Model file for the job. Use its own axes, mm. Round coordinates to 2 decimals unless told otherwise and drop trailing zeros. Write each loop counter-clockwise with the first axis right and the second up, starting at its lowest first coordinate (ties: lowest second). Pieces come first, ordered by that corner, then holes. Notation, with made-up numbers: (-26.75, 43.5) - (15.25, 43.5) arc R24 ccw to (15.25, 67.5) - close; hole circle Ø8 at (23.25, -29.75). An arc over 180 degrees is marked (long way). Answer as a JSON object with one key per item and string values. Group by question number.
from build123d import *

# Parameters (mm, degrees)
SKETCH_1_R          = 1.9
EXTRUDE_1_DEPTH     = 72
SKETCH_2_R          = 2.25
CUT_EXTRUDE_1_DEPTH = 2.1


with BuildPart() as part:
    # 草图1 → 凸台-拉伸1 (new body)
    with BuildSketch(Plane(origin=(0, 0, 0), x_dir=(0, 0, -1), z_dir=(1, 0, 0))):
        with Locations((22, 3)):
            Circle(SKETCH_1_R)
        with BuildLine():
            Line((0, 1.1), (0, 0))
            Line((0, 0), (19, 0))
            Line((19, 0), (23.9, 0))
            Line((23.9, 0), (23.9, 3))
            ThreePointArc((23.9, 3), (23.343502884, 1.656497116), (22, 1.1))
            Line((22, 1.1), (19, 1.1))
            Line((19, 1.1), (0, 1.1))
        make_face()
    extrude(amount=EXTRUDE_1_DEPTH)

    # 草图2 → 切除-拉伸1 (cut, through all)
    with BuildSketch(Plane(origin=(0, 1.1, 0), x_dir=(1, 0, 0), z_dir=(0, 1, 0))):
        with Locations((8.15, 8.15)):
            Circle(SKETCH_2_R)
        with Locations((63.85, 8.15)):
            Circle(SKETCH_2_R)
    extrude(amount=-CUT_EXTRUDE_1_DEPTH, mode=Mode.SUBTRACT)


solid = part.part
(1) Slice it at A-A (x = 8.15). Write the cut outline in (y, z), then the cut area to 3 significant figures.
(2) Slice it at D-D (z = -13.75). Write the cut outline in (x, y).
(3) Slice it at B-B (z = -21). Write the cut outline in (x, y), then the cut area to 3 significant figures.
(4) Flat gauge pins, fed straight in: pin 1 (10 mm diameter, centred on x = 25, z = -8, fed in from +Y); pin 2 (5 mm diameter, centred on x = 63.85, z = -8.15, fed in from -Y); pin 3 (2 mm diameter, centred on y = 3, z = -10, fed in from +X). Where does each tip first touch, or does it go through?
(5) Slice it at C-C (x = 55.5). Write the cut outline in (y, z).
(6) Pull direction Y, two halves, no side cores. Call faces 1 (the flat face through (35, 0, -12)), 2 (the cylindrical face through (35.496, 4.387, -20.702)), 3 (the flat face through (0, 0.8, -15.4)): pulls with the +Y half, pulls with the -Y half, needs draft (parallel to the pull), parting line crosses it, or undercut.
(7) Drill centre lines: line 1 (X direction, y = 0.3, z = -8.15); line 2 (Z direction, x = 8, y = 0.85) (3 decimals); line 3 (Y direction, x = 15, z = -10). Where is each one in solid material? Low to high. Write a range as from..to.
Answer:
{
 "1": {"outline": "(0, -23.9) - (3, -23.9) arc R1.9 ccw (long way) to (1.1, -22) - (1.1, -10.4) - (0, -10.4) - close; (0, -5.9) - (1.1, -5.9) - (1.1, 0) - (0, 0) - close", "area": "33.5 mm²"},
 "2": {"outline": "(0, 0) - (72, 0) - (72, 1.1) - (0, 1.1) - close"},
 "3": {"outline": "(0, 0) - (72, 0) - (72, 1.1) - (0, 1.1) - close; (0, 1.38) - (72, 1.38) - (72, 4.62) - (0, 4.62) - close", "area": "312 mm²"},
 "4": {"pin 1": "y = 1.1", "pin 2": "y = 0", "pin 3": "through"},
 "5": {"outline": "(0, -23.9) - (3, -23.9) arc R1.9 ccw (long way) to (1.1, -22) - (1.1, 0) - (0, 0) - close"},
 "6": {"face 1": "pulls with the -Y half", "face 2": "undercut", "face 3": "needs draft"},
 "7": {"line 1": "0..5.9, 10.4..61.6, 66.1..72", "line 2": "-23.9..-10.395, -5.905..0", "line 3": "0..1.1"}
}
